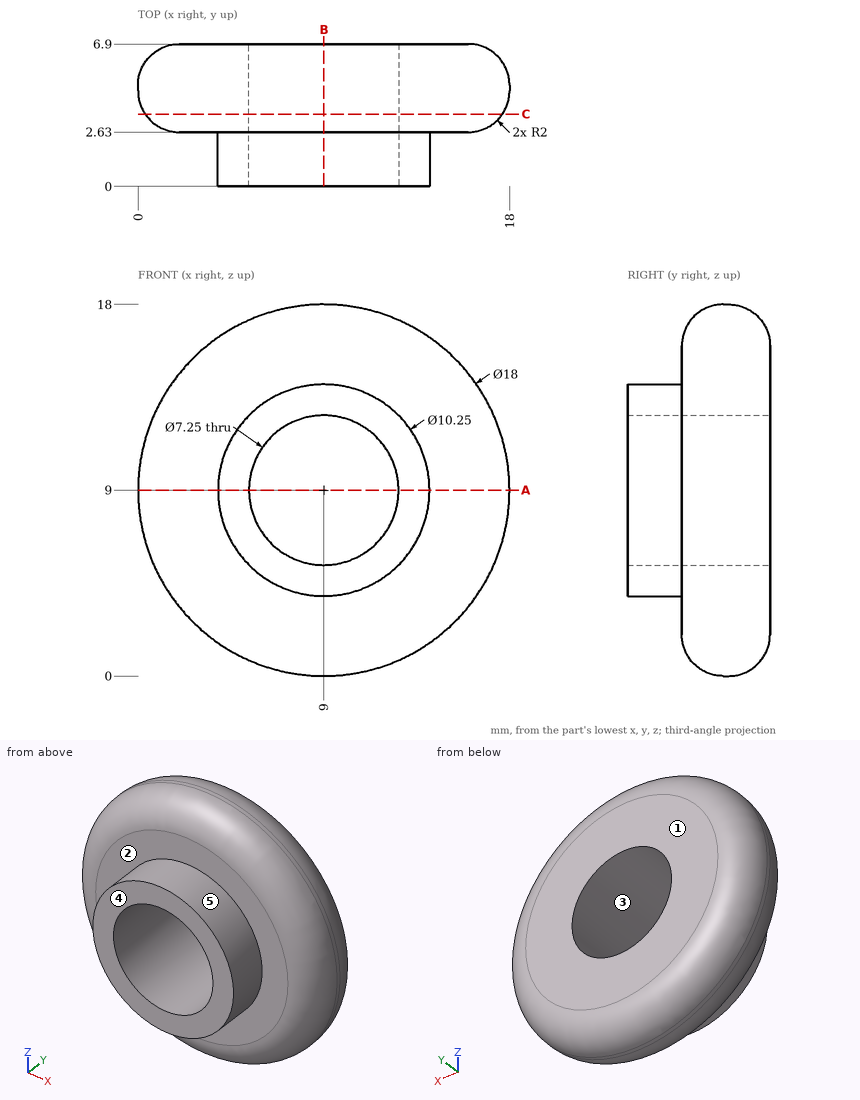
Job drawing, mm, ordinate dimensions from the low corner. One solid piece. A direction names the side the tool comes from. Round coordinates to 2 decimals unless told otherwise and drop trailing zeros. Loops run counter-clockwise (first coordinate to the right, second up) from the corner with the lowest first, then second, coordinate; pieces in that order, holes last. Notation, with made-up numbers: (23.5, 6.25) -> (75.5, 6.25) arc R25 cw to (75.5, 25.25) -> close; hole circle Ø11 at (2, -38). An arc over 180 degrees is marked (long way). Use CSV: the item, a comma, the result in double quotes. Start each with the question number.
Q1. Which spindle directions (+Z, -Z, +X, -X, +Y, -Y) get a long thin tool onto all of the face, cutting with end or side? Do the marked faces 1 and 2. Say none if no direction does.
Q2. Saw through at B-B on x = 9. Give the cut face in (y, z) (3 decimals), and give its area (3 significant figures).
Q3. Saw through at C-C on y = 3.5. Give the cut face in (x, z) (3 decimals), and give its area (3 significant figures).
Q4. Saw through at A-A on z = 9. Give the cut face in (x, y) (3 decimals).
Q5. Mould opens along Z. For the marked faces 3, 4 and 5 say: +Z half, -Z half, draft (parallel to the pull), parting line (faces both ways), or undercut.
Q6. Flat gauge pins, fed straight in: pin 1 Ø6 at (x, z) = (9, 9) entering from +Y; pin 2 Ø2 at (y, z) = (1, 14) entering from +X; pin 3 Ø1 at (x, y) = (12, 5) entering from -Z; pin 4 Ø1.5 at (y, z) = (1.5, 14) entering from +X. Where does each tip first touch, or does it go through?
Q7. Drill centre lines: L1, parallel to Z at x = 9, y = 2 (3 decimals); L2, parallel to Z at x = 9, y = 4.75 (3 decimals); L3, parallel to Y at x = 4.25, z = 14. Where is each one in solid material? Low to high.
Solutions:
1,face 1,"+Z, -Z, +X, -X, +Y"
1,face 2,"-Y"
2,outline,"(0, 3.875) -> (2.63, 3.875) -> (2.63, 2) arc R2 ccw to (4.63, 0) -> (4.9, 0) arc R2 ccw to (6.9, 2) -> (6.9, 5.375) -> (0, 5.375) -> close; (0, 12.625) -> (6.9, 12.625) -> (6.9, 16) arc R2 ccw to (4.9, 18) -> (4.63, 18) arc R2 ccw to (2.63, 16) -> (2.63, 14.125) -> (0, 14.125) -> close"
2,area,"50.4 mm^2"
3,outline,"circle Ø17.3 at (9, 9); hole circle Ø7.25 at (9, 9)"
3,area,"194 mm^2"
4,outline,"(0, 4.63) arc R2 ccw to (2, 2.63) -> (3.875, 2.63) -> (3.875, 0) -> (5.375, 0) -> (5.375, 6.9) -> (2, 6.9) arc R2 ccw to (0, 4.9) -> close; (12.625, 0) -> (14.125, 0) -> (14.125, 2.63) -> (16, 2.63) arc R2 ccw to (18, 4.63) -> (18, 4.9) arc R2 ccw to (16, 6.9) -> (12.625, 6.9) -> close"
5,face 3,"undercut"
5,face 4,"draft"
5,face 5,"parting line"
6,pin 1,"passes through"
6,pin 2,"stops at x = 12.2"
6,pin 3,"stops at z = 0.36"
6,pin 4,"stops at x = 11.86"
7,L1,"z = 3.875 to 5.375, 12.625 to 14.125"
7,L2,"z = 0 to 5.375, 12.625 to 18"
7,L3,"y = 2.63 to 6.9"
